Verification items for the finished model (mm, model axes). Face numbers are marked on the shaded views. A direction names the side the tool comes from. Round coordinates to 2 decimals unless told otherwise and drop trailing zeros. Write each loop counter-clockwise with the first axis right and the second up, starting at its lowest first coordinate (ties: lowest second). Pieces come first, ordered by that corner, then holes. Notation, with made-up numbers: M 2.25,-1.5 L 56.25,-1.5 A9 ccw 56.25,9.5 Z; hole C 63,6.5 d2. An arc over 180 degrees is marked long. One line per question, with ' | ' between items. Start each with the question number.
Q1. Thickness scan on line 1 along Z through (x, y) = (7, -17); line 2 along Z through (x, y) = (-16, 34); line 3 along Y through (x, z) = (-37, 14.5). Record the ranges inside material, lowest first. Write a range as from..to.
Q2. Gauge pin test, flat ends, axial feed: pin 1 (10 mm diameter, centred on x = -14, z = 24.5, fed in from -Y); pin 2 (4 mm diameter, centred on x = -27.5, y = -21, fed in from +Z); pin 3 (12 mm diameter, centred on y = -9, z = 7, fed in from -X); pin 4 (8 mm diameter, centred on y = -35.5, z = 30.5, fed in from -X). Record the tip position at first contact, or that the pin passes through.
Q3. Cross-section at D-D (z = 8.5). Record the boundary of the cut face in (x, y), then the cut area to 3 significant figures.
Q4. Cross-section at C-C (z = 25.5). Record the boundary of the cut face in (x, y), then the cut area to 3 significant figures.
Q5. Release check for a two-part mould opening along Z. For the marked faces 1, 2 and 3 record: released by +Z, released by -Z, zero draft, split by the parting line, or undercut.
Q6. Cross-section at A-A (x = 0). Record the boundary of the cut face in (y, z), then the cut area to 3 significant figures.
Q7. Tool access check on the marked faces 4, 5 and 6. Record the directions out of +Z, -Z, +X, -X, +Y, -Y that give a thin tool (end or side, any length) a straight path to the whole face; none if there is none.
from build123d import *

# Parameters (mm, degrees)
ESQUISSE1_R        = 45
BOSS_EXTRU_1_DEPTH = 15
ESQUISSE3_R        = 10
BOSS_EXTRU_2_DEPTH = 20
ESQUISSE4_R        = 30
BOSS_EXTRU_3_DEPTH = 10
CONG_1_R           = 2
CONG_2_R           = 1
CONG_3_R           = 1


with BuildPart() as part:
    # Esquisse1 → Boss.-Extru.1 (new body)
    with BuildSketch(Plane.XY):
        Circle(ESQUISSE1_R)
    extrude(amount=BOSS_EXTRU_1_DEPTH)

    # Esquisse3 → Boss.-Extru.2 (add)
    with BuildSketch(Plane.XY.offset(15)):
        Circle(ESQUISSE3_R)
    extrude(amount=BOSS_EXTRU_2_DEPTH)

    # Esquisse4 → Boss.-Extru.3 (add)
    with BuildSketch(Plane.XY.offset(35)):
        Circle(ESQUISSE4_R)
    extrude(amount=BOSS_EXTRU_3_DEPTH)

    # Congé1
    cong_1_edges = [part.edges().sort_by_distance(p)[0] for p in [
        (-45, 0, 15),
    ]]
    fillet(cong_1_edges, radius=CONG_1_R)

    # Congé2
    cong_2_edges = [part.edges().sort_by_distance(p)[0] for p in [
        (-30, 0, 35),
    ]]
    fillet(cong_2_edges, radius=CONG_2_R)

    # Congé3
    cong_3_edges = [part.edges().sort_by_distance(p)[0] for p in [
        (-45, 0, 0),
    ]]
    fillet(cong_3_edges, radius=CONG_3_R)


solid = part.part
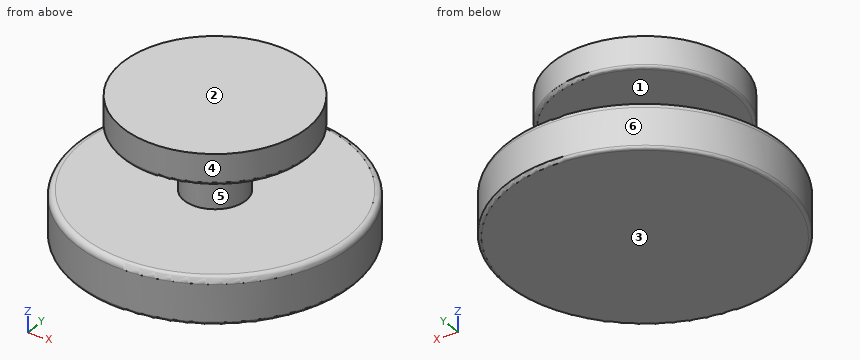
Determined:
1) line 1: z = 0..15, 35..45 | line 2: z = 0..15 | line 3: y = -24.4..24.4
2) pin 1: stops at y = -4.36 | pin 2: stops at z = 15 | pin 3: stops at x = -44.9 | pin 4: passes through
3) outline: C 0,0 d90 | area: 6,360 mm²
4) outline: C 0,0 d20 | area: 314 mm²
5) face 1: undercut | face 2: released by +Z | face 3: released by -Z
6) outline: M -45,1 A1 ccw -44,0 L 44,0 A1 ccw 45,1 L 45,13 A2 ccw 43,15 L 10,15 L 10,35 L 29,35 A1 ccw 30,36 L 30,45 L -30,45 L -30,36 A1 ccw -29,35 L -10,35 L -10,15 L -43,15 A2 ccw -45,13 Z | area: 2,350 mm²
7) face 4: +Z | face 5: none | face 6: +Z, -Z
